The listing builds one solid part. Answer for the finished solid, in the listing's coordinates (mm). Face numbers are marked on the shaded views. A direction names the side the tool comes from. Coordinates: 2 decimals unless noted, no trailing zeros. Loops run counter-clockwise (first coordinate to the right, second up) from the corner with the lowest first, then second, coordinate; pieces in that order, holes last. Notation, with made-up numbers: (-34.5, 80) - (13.5, 80) arc R21 cw to (13.5, 85) - close; hole circle Ø8 at (34, -38.5). An arc over 180 degrees is marked (long way). One line per question, with ' | ' between items.
Autodesk Inventor part; units mm, degrees
ref_plane "YZ Plane" through (0, 0, 0) normal (1, 0, 0) x (0, 1, 0)
ref_plane "XZ Plane" through (0, 0, 0) normal (0, 1, 0) x (-1, 0, 0)
ref_plane "XY Plane" through (0, 0, 0) normal (0, 0, 1) x (1, 0, 0)
sketch "스케치1" plane through (0, 0, 0) normal (0, 0, 1) x (1, 0, 0)
  line L0 (0, 0) -> (16, 0)
  line L1 (16, 48) -> (0, 48)
  line L2 (0, 48) -> (0, 0)
  line L3 (0, 0) -> (20, 0)
  line L4 (0, 0) -> (20, 0) construction
  circle A0 centre (20, 5) radius 2
  line L5 (20, 10) -> (16, 10)
  circle A1 centre (20, 5) radius 5
  line L6 (16, 48) -> (16, 10)
  circle A2 centre (8, 40) radius 4
  line L7 (4, 16) -> (12, 16)
  line L8 (12, 16) -> (12, 4)
  line L9 (12, 4) -> (4, 4)
  line L10 (4, 4) -> (4, 16)
  line L11 (0, 25) -> (16, 25)
  dimension "d0" = 16
  dimension "d4" = 48
  dimension "d5" = 20
  dimension "d8" = 4
  dimension "d9" = 10
  dimension "d10" = 8
  dimension "d11" = 40
  dimension "d12" = 8
  dimension "d13" = 12
  dimension "d14" = 4
  dimension "d15" = 4
  dimension "d16" = 8
  dimension "d17" = 25
extrude "돌출1" add sketch "스케치1" against normal blind 6.5 contours L2 L11 L6 L5 A1 L3 L0 | A1
extrude "돌출2" add sketch "스케치1" along normal mid plane 13 contours L2 L1 L6 L11
fillet "모깎기1" radius 8 2 edges at (16, 48, 0) (0, 48, 0)
fillet "모깎기2" radius 3 4 edges at (4, 16, -3.25) (12, 16, -3.25) (12, 4, -3.25) (4, 4, -3.25)
fillet "모깎기3" radius 8 1 edges at (16, 10, -3.25)
sketch "스케치2" plane through (0, 0, 0) normal (0, 0, 1) x (1, 0, 0)
  line L0 (-9.7469, 60.6249) -> (29.3105, 60.6249)
  line L1 (29.3105, 60.6249) -> (29.3105, 31)
  line L2 (29.3105, 31) -> (-9.7469, 31)
  line L3 (-9.7469, 31) -> (-9.7469, 60.6249)
  point P0 (0, 0)
  dimension "d25" = 31
extrude "돌출3" cut sketch "스케치2" along normal mid plane 6
properties part number "2번부품"
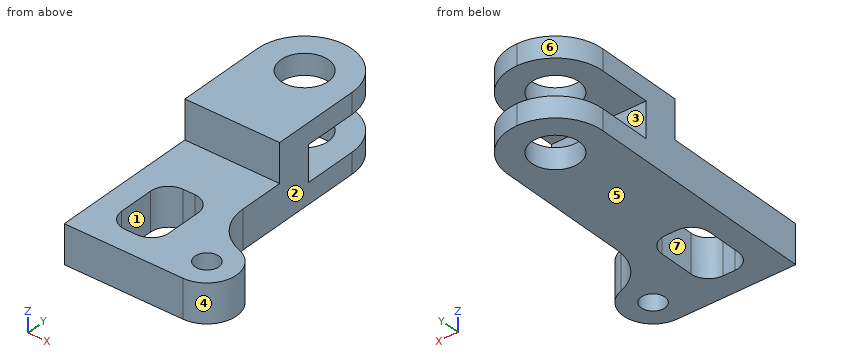
Item 1: Which of the six approach directions +Z, -Z, +X, -X, +Y, -Y give full straight-line access (tool end or side, diameter ignored) to the marked faces 1, 2 and 3?
Taken from the geometry:
face 1: +Z, -Z | face 2: +Z, -Z, +X, +Y | face 3: +X, -X, +Y
Item 2: Each of these flat-tipped pins is pushed along its axis until it touches: pin 1 Ø2 at (x, z) = (4.5, 4) entering from -Y; pin 2 Ø5 at (y, z) = (9.5, -2.5) entering from +X; pin 3 Ø1.6 at (x, z) = (8, -2) entering from +Y. Where does it stop, or does it pass through?
Taken from the geometry:
pin 1: stops at y = 25 | pin 2: stops at x = 24.58 | pin 3: stops at y = 31
Item 3: Find section B-B, the plane y = 5. Write down the section's boundary in (x, z), plus the area to 3 significant figures.
Taken from the geometry:
outline: (0, -6.5) - (4.76, -6.5) - (4.76, 0) - (0, 0) - close; (11.24, -6.5) - (18, -6.5) - (18, 0) - (11.24, 0) - close; (22, -6.5) - (25, -6.5) - (25, 0) - (22, 0) - close | area: 94.4 mm2
Item 4: The mould has two halves that part along X. Classify the marked faces 4, 5, 6 and 7: pulls with the +X half, pulls with the -X half, needs draft (parallel to the pull), parting line crosses it, or undercut.
Taken from the geometry:
face 4: pulls with the +X half | face 5: needs draft | face 6: pulls with the -X half | face 7: undercut
Item 5: Find section C-C, the plane y = 43. Write down the section's boundary in (x, z).
Taken from the geometry:
outline: (0.58, -6.5) - (5.35, -6.5) - (5.35, -3) - (0.58, -3) - close; (0.58, 3) - (5.35, 3) - (5.35, 6.5) - (0.58, 6.5) - close; (10.65, -6.5) - (15.42, -6.5) - (15.42, -3) - (10.65, -3) - close; (10.65, 3) - (15.42, 3) - (15.42, 6.5) - (10.65, 6.5) - close
Item 6: Find section D-D, the plane z = -3.5. State how many separate pieces and enclosed holes the cut face has, plus the area to 3 significant figures.
Taken from the geometry:
separate pieces: 1 | enclosed holes: 3 | area: 679 mm2
Item 7: Find the intervals of material crossed by line 1 (Y direction, x = 8, z = -5.5); line 2 (X direction, y = 40, z = -4); line 3 (Z direction, x = 7, y = 35.5), in increasing order. Write a range as [from, to].
Taken from the geometry:
line 1: y = [0, 4], [16, 36], [44, 48] | line 2: x = [0, 4], [12, 16] | line 3: z = [-6.5, -3], [3, 6.5]
Item 8: Find section A-A, the plane x = 10.5. Write down the section's boundary in (y, z).
Taken from the geometry:
outline: (0, -6.5) - (4.4, -6.5) - (4.4, 0) - (0, 0) - close; (15.6, -6.5) - (36.88, -6.5) - (36.88, -3) - (31, -3) - (31, 3) - (36.88, 3) - (36.88, 6.5) - (25, 6.5) - (25, 0) - (15.6, 0) - close; (43.12, -6.5) - (47.6, -6.5) - (47.6, -3) - (43.12, -3) - close; (43.12, 3) - (47.6, 3) - (47.6, 6.5) - (43.12, 6.5) - close
